Study the drawing (mm; zero at the part's minimum x, y, z) and answer. Round coordinates to 2 decimals unless told otherwise and drop trailing zeros. Loops run counter-clockwise (first coordinate to the right, second up) from the corner with the lowest first, then second, coordinate; pieces in that order, holes last. Notation, with made-up numbers: (16.5, -9.5) -> (31.5, -9.5) arc R27 ccw to (31.5, 24.5) -> close; hole circle Ø7 at (56, -27.75). An arc over 180 degrees is marked (long way). Use one line per item in the form item = value.
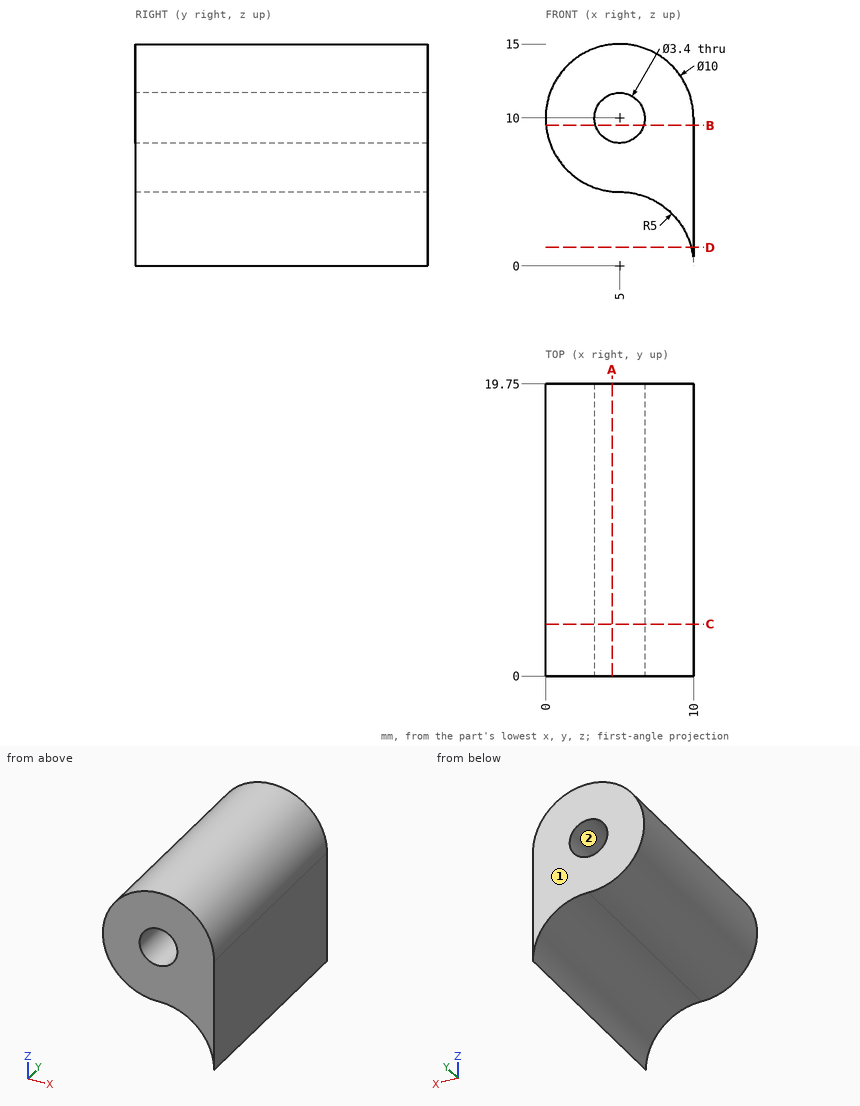
(1) Find section C-C, the plane y = 3.5. Write down the section's boundary in (x, z), then the cut area to 3 significant figures.
Completed:
outline = (5, 5) arc R5 cw to (10, 0) -> (10, 10) arc R5 ccw (long way) to start; hole circle Ø3.4 at (5, 10)
area = 80.2 mm2
(2) Consider L1, parallel to X at y = 13.75, z = 10; L2, parallel to X at y = 2.5, z = 10.75; L3, parallel to Z at x = 4.75, y = 17.75. Determine where each line is inside the solid, lowest interval first.
Completed:
L1 = 0 to 3.3, 6.7 to 10
L2 = 0.06 to 3.47, 6.53 to 9.94
L3 = 5.01 to 8.32, 11.68 to 14.99
(3) Find section B-B, the plane z = 9.5. Write down the section's boundary in (x, y).
Completed:
outline = (0.03, 0) -> (3.38, 0) -> (3.38, 19.75) -> (0.03, 19.75) -> close; (6.62, 0) -> (10, 0) -> (10, 19.75) -> (6.62, 19.75) -> close
(4) Given P1, Ø2, axis at x = 4.5, y = 17.5, coming from the -Z side; P2, Ø3, axis at y = 11.5, z = 7.5, coming from the -X side; P3, Ø2, axis at x = 1, y = 16.5, coming from the +Z side, each flat-ended and moving along its own axis, determine where each tip first touches the part or whether it passes through.
Completed:
P1 = 4.97
P2 = 0.1
P3 = 14
(5) For a pull along Z with two mould halves and no side action, classify the marked faces 1 and 2 as +Z half, -Z half, draft (parallel to the pull), parting line (faces both ways), or undercut.
Completed:
face_1 = draft
face_2 = undercut
(6) Find section D-D, the plane z = 1.25. Write down the section's boundary in (x, y), then the cut area to 3 significant figures.
Completed:
outline = (9.84, 0) -> (10, 0) -> (10, 19.75) -> (9.84, 19.75) -> close
area = 3.14 mm2
(7) Find section A-A, the plane x = 4.5. Write down the section's boundary in (y, z), then the cut area to 3 significant figures.
Completed:
outline = (0, 5.03) -> (19.75, 5.03) -> (19.75, 8.38) -> (0, 8.38) -> close; (0, 11.62) -> (19.75, 11.62) -> (19.75, 14.97) -> (0, 14.97) -> close
area = 132 mm2
